Model file for the job. Use its own axes, mm. A direction names the side the tool comes from. Give positions to 0.01 mm unless a question says otherwise; leave off trailing zeros. Loops run counter-clockwise (first coordinate to the right, second up) from the corner with the lowest first, then second, coordinate; pieces in that order, holes last. Notation, with made-up numbers: (16.25, 44) - (69.25, 44) arc R19 ccw to (69.25, 57) - close; hole circle Ø6 at (42, -4). An arc over 180 degrees is marked (long way). Answer as CSV lines item,"result". Start each with the question number.
Item 1: Saw through at D-D on z = 8. Give the cut face in (x, y).
Item 2: Drill centre lines: L1, parallel to Y at x = 0, z = 13; L2, parallel to X at y = -24.5, z = 29; L3, parallel to X at y = -31.5, z = 18.05. Where is each one in solid material? Low to high. Write a range as from..to.
Item 3: Pin check, flat tips, straight feed: pin 1 (4 mm diameter, centred on x = -3, y = -10.5, fed in from -Z); pin 2 (10 mm diameter, centred on x = 6, z = 32, fed in from +Y); pin 3 (6 mm diameter, centred on x = 7.5, z = 14.5, fed in from +Y); pin 4 (13.5 mm diameter, centred on x = 0, y = -40, fed in from -Z). Stop position of each tip, or through.
Item 4: Saw through at A-A on z = 18. Give the cut face in (x, y).
Item 5: Saw through at B-B on y = 31.5. Give the cut face in (x, z), plus the area to 3 significant figures.
Item 6: Saw through at C-C on x = -2.5. Give the cut face in (y, z), plus the area to 3 significant figures.
Item 7: Tool access for faces 1 (the flat face through (0, 27.5, 30)), 2 (the cylindrical face through (0.94, -47.19, 7.64)), 3 (the flat face through (0, -30, 30)): list every direction of +Z, -Z, +X, -X, +Y, -Y with a clear straight run to the whole face (end or side of a thin tool).
Item 8: Pull direction Y, two halves, no side cores. Call faces 4 (the cylindrical face through (9.92, -37.96, 17.54)), 5 (the flat face through (-12.5, 0, 30)), 6 (the cylindrical face through (-1.96, -36.23, 9.86)), 7 (the cylindrical face through (10.04, 37.86, 17.54)): pulls with the +Y half, pulls with the -Y half, needs draft (parallel to the pull), parting line crosses it, or undercut.
from build123d import *

# Parameters (mm, degrees)
ESBO_O1_R                  = 7.25
ESBO_O1_R_2                = 4.25
RESSALTO_EXTRUS_O1_DEPTH   = 20
RESSALTO_EXTRUS_O1_2_DEPTH = 20
ESBO_O2_W                  = 30
ESBO_O2_H                  = 71.5
RESSALTO_EXTRUS_O2_DEPTH   = 5
FILETE1_R                  = 10
ESBO_O3_W                  = 30
ESBO_O3_H                  = 60
ESBO_O3_W_2                = 25
ESBO_O3_H_2                = 55
RESSALTO_EXTRUS_O3_DEPTH   = 20
ESBO_O4_R                  = 1
CORTE_EXTRUS_O1_DEPTH      = 54.456173638


with BuildPart() as part:
    # Esbo_o1 → Ressalto-extrus_o1 (new body)
    with BuildSketch(Plane.XY):
        with Locations((0, 40)):
            Circle(ESBO_O1_R)
        with Locations((0, 40)):
            Circle(ESBO_O1_R_2, mode=Mode.SUBTRACT)
    extrude(amount=RESSALTO_EXTRUS_O1_DEPTH)



with BuildPart() as body_2:
    # Esbo_o1 → Ressalto-extrus_o1 2 (new body)
    with BuildSketch(Plane.XY):
        with Locations(Location((0, -40, 0), (0, 0, 180))):
            Circle(ESBO_O1_R)
        with Locations(Location((0, -40, 0), (0, 0, 180))):
            Circle(ESBO_O1_R_2, mode=Mode.SUBTRACT)
    extrude(amount=RESSALTO_EXTRUS_O1_2_DEPTH)


with BuildPart() as part_1:
    add(part.part)

    add(body_2.part)  # Ressalto-extrus_o2 merges body 2
    # Esbo_o2 → Ressalto-extrus_o2 (add)
    with BuildSketch(Plane.XY.offset(20)):
        Rectangle(ESBO_O2_W, ESBO_O2_H)
    extrude(amount=-RESSALTO_EXTRUS_O2_DEPTH)

    # Filete1
    # the kernel refuses this fillet: 10 mm, written as the material it adds along each edge
    with BuildSketch(Plane(origin=(-5.873670062, -35.75, 20), x_dir=(-1, 0, 0), z_dir=(0, 0, -1))) as filete1_piece_1:
        with BuildLine():
            CenterArc((10.419216441, -9.916070012), FILETE1_R, 97.428488086, 63.395706738)
            Line((0.974064845, -6.631391744), (0.785161813, -6.565698179))
            ThreePointArc((0.785161813, -6.565698179), (1.101484321, -3.225440913), (-0.162032278, -0.117241379))
            Line((-0.162032278, -0.117241379), (0, 0.2))
            ThreePointArc((0, 0.2), (4.563164969, 0.2), (9.100472208, 0.1983214))
            Line((9.100472208, 0.1983214), (9.126329938, 0))
        make_face()
    extrude(amount=5)
    with BuildSketch(Plane(origin=(5.873670062, -35.75, 20), x_dir=(1, 0, 0), z_dir=(0, 0, -1))) as filete1_piece_2:
        with BuildLine():
            CenterArc((10.419216441, 9.916070012), FILETE1_R, 199.175805176, 63.395706738)
            Line((0.974064845, 6.631391744), (0.785161813, 6.565698179))
            ThreePointArc((0.785161813, 6.565698179), (1.101484321, 3.225440913), (-0.162032278, 0.117241379))
            Line((-0.162032278, 0.117241379), (0, -0.2))
            ThreePointArc((0, -0.2), (4.563164969, -0.2), (9.100472208, -0.1983214))
            Line((9.100472208, -0.1983214), (9.126329938, 0))
        make_face()
    extrude(amount=5)
    with BuildSketch(Plane(origin=(5.873670062, 35.75, 20), x_dir=(0.14532753012910826, 0.9893836005243736, 0), z_dir=(0, 0, -1))) as filete1_piece_3:
        with BuildLine():
            CenterArc((11.324996043, 8.867523914), FILETE1_R, 179.072241898, 63.395706738)
            Line((1.326306989, 9.029441173), (1.126333208, 9.032679519))
            ThreePointArc((1.126333208, 9.032679519), (0.465276774, 4.543786093), (-0.19787672, 0.029065506))
            Line((-0.19787672, 0.029065506), (0.092448947, -0.177350478))
            ThreePointArc((0.092448947, -0.177350478), (3.351274339, 0.621045162), (6.610099731, -0.177350478))
            Line((6.610099731, -0.177350478), (6.702548679, 0))
        make_face()
    extrude(amount=5)
    with BuildSketch(Plane(origin=(-5.873670062, 35.75, 20), x_dir=(-0.14532753012910826, 0.9893836005243736, 0), z_dir=(0, 0, -1))) as filete1_piece_4:
        with BuildLine():
            CenterArc((11.324996043, -8.867523914), FILETE1_R, 117.532051364, 63.395706738)
            Line((1.326306989, -9.029441173), (1.126333208, -9.032679519))
            ThreePointArc((1.126333208, -9.032679519), (0.465276774, -4.543786093), (-0.19787672, -0.029065506))
            Line((-0.19787672, -0.029065506), (0.092448947, 0.177350478))
            ThreePointArc((0.092448947, 0.177350478), (3.351274339, -0.621045162), (6.610099731, 0.177350478))
            Line((6.610099731, 0.177350478), (6.702548679, 0))
        make_face()
    extrude(amount=5)

    # Esbo_o3 → Ressalto-extrus_o3 (add)
    with BuildSketch(Plane.XY.offset(20)):
        Rectangle(ESBO_O3_W, ESBO_O3_H)
        Rectangle(ESBO_O3_W_2, ESBO_O3_H_2, mode=Mode.SUBTRACT)
    extrude(amount=RESSALTO_EXTRUS_O3_DEPTH)

    # Esbo_o4 → Corte-extrus_o1 (cut, through all)
    with BuildSketch(Plane.XY.offset(20)):
        with Locations((0, 31.5)):
            Circle(ESBO_O4_R)
        with Locations(Location((0, -31.5, 0), (0, 0, 180))):
            Circle(ESBO_O4_R)
    extrude(amount=-CORTE_EXTRUS_O1_DEPTH, mode=Mode.SUBTRACT)


solid = part_1.part
Responses:
1,outline,"circle Ø14.5 at (0, -40); circle Ø14.5 at (0, 40); hole circle Ø8.5 at (0, -40); hole circle Ø8.5 at (0, 40)"
2,L1,"-47.25..-44.25, -35.75..-32.75, 32.75..35.75, 44.25..47.25"
2,L2,"-15..-12.5, 12.5..15"
2,L3,"-15..-1, 1..15"
3,pin 1,"z = 15"
3,pin 2,"y = 30"
3,pin 3,"y = 45.68"
3,pin 4,"z = 0"
4,outline,"(-15, -35.75) arc R10 cw to (-6.85, -42.38) arc R7.25 ccw to (6.85, -42.38) arc R10 cw to (15, -35.75) - (15, 35.75) arc R10 cw to (6.85, 42.38) arc R7.25 ccw to (-6.85, 42.38) arc R10 cw to (-15, 35.75) - close; hole circle Ø8.5 at (0, -40); hole circle Ø8.5 at (0, 40); hole circle Ø2 at (0, -31.5); hole circle Ø2 at (0, 31.5)"
5,outline,"(-15, 15) - (-1, 15) - (-1, 20) - (-15, 20) - close; (1, 15) - (15, 15) - (15, 20) - (1, 20) - close"
5,area,"140 mm2"
6,outline,"(-46.81, 0) - (-43.44, 0) - (-43.44, 20) - (-46.81, 20) - close; (-36.56, 0) - (-33.19, 0) - (-33.19, 15) - (33.19, 15) - (33.19, 0) - (36.56, 0) - (36.56, 20) - (30, 20) - (30, 40) - (27.5, 40) - (27.5, 20) - (-27.5, 20) - (-27.5, 40) - (-30, 40) - (-30, 20) - (-36.56, 20) - close; (43.44, 0) - (46.81, 0) - (46.81, 20) - (43.44, 20) - close"
6,area,"701 mm2"
7,face 1,"+Z"
7,face 2,"-Z"
7,face 3,"+Z, +X, -X, -Y"
8,face 4,"pulls with the -Y half"
8,face 5,"undercut"
8,face 6,"undercut"
8,face 7,"pulls with the +Y half"
